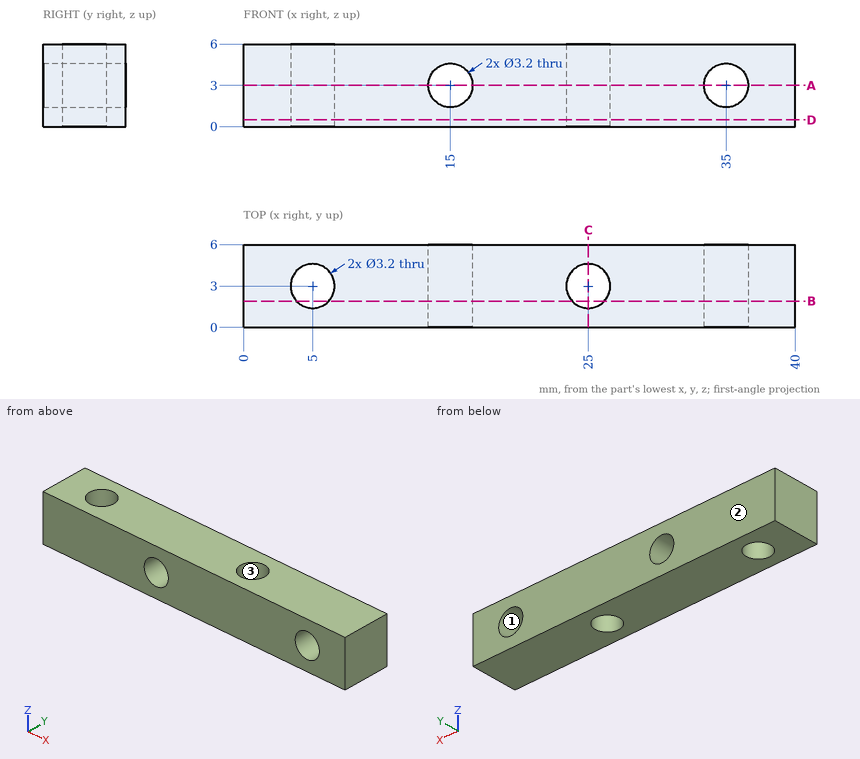
Verification items for this drawing (mm, ordinates from the low corner). Coordinates: 2 decimals unless noted, no trailing zeros. Loops run counter-clockwise (first coordinate to the right, second up) from the corner with the lowest first, then second, coordinate; pieces in that order, holes last. Notation, with made-up numbers: (66.25, 61.5) - (90.25, 61.5) arc R19 ccw to (90.25, 94.5) - close; hole circle Ø6 at (43, 45). An arc over 180 degrees is marked (long way). Use one line per item in the form item = value. Start each with the question number.
Item 1: Section check A-A, the plane z = 3. Enter the section's corners in (x, y).
Item 2: Mould release check, pull along Y, two halves, no side actions. Record for the marked faces 1, 2 and 3: +Y half, -Y half, draft (parallel to the pull), parting line (faces both ways), or undercut.
Item 3: Section check B-B, the plane y = 1.9. Enter the section's corners in (x, z), and give its area (3 significant figures).
Item 4: Section check D-D, the plane z = 0.5. Enter the section's corners in (x, y), and give its area (3 significant figures).
Item 5: Section check C-C, the plane x = 25. Enter the section's corners in (y, z), and give its area (3 significant figures).
Item 6: Thickness scan on probe 1 along Z at (x, y) = (35, 4.2); probe 2 along X at (y, z) = (3.9, 1.1); probe 3 along X at (y, z) = (4.7, 2.7). Record the ranges inside material, lowest first.
Computed:
q1.outline = (0, 0) - (13.4, 0) - (13.4, 6) - (0, 6) - close; (16.6, 0) - (33.4, 0) - (33.4, 6) - (16.6, 6) - close; (36.6, 0) - (40, 0) - (40, 6) - (36.6, 6) - close; hole circle Ø3.2 at (5, 3); hole circle Ø3.2 at (25, 3)
q2.face_1 = draft
q2.face_2 = +Y half
q2.face_3 = undercut
q3.outline = (0, 0) - (3.84, 0) - (3.84, 6) - (0, 6) - close; (6.16, 0) - (23.84, 0) - (23.84, 6) - (6.16, 6) - close; (26.16, 0) - (40, 0) - (40, 6) - (26.16, 6) - close; hole circle Ø3.2 at (15, 3); hole circle Ø3.2 at (35, 3)
q3.area = 196 mm2
q4.outline = (0, 0) - (40, 0) - (40, 6) - (0, 6) - close; hole circle Ø3.2 at (5, 3); hole circle Ø3.2 at (25, 3)
q4.area = 224 mm2
q5.outline = (0, 0) - (1.4, 0) - (1.4, 6) - (0, 6) - close; (4.6, 0) - (6, 0) - (6, 6) - (4.6, 6) - close
q5.area = 16.8 mm2
q6.probe_1 = 0 to 1.4, 4.6 to 6
q6.probe_2 = 0 to 3.68, 6.32 to 23.68, 26.32 to 40
q6.probe_3 = 0 to 13.43, 16.57 to 33.43, 36.57 to 40
